```python
from build123d import *

# Parameters (mm, degrees)
BOSS_EXTRUDE1_DEPTH = 3.2
SKETCH2_R           = 6
CUT_EXTRUDE1_DEPTH  = 10


with BuildPart() as part:
    # Sketch1 → Boss-Extrude1 (new body)
    with BuildSketch(Plane.XY):
        with BuildLine():
            ThreePointArc((2.3749, 17.446481614), (2.211827147, 19.125468185), (1.72870442, 20.741692518))
            ThreePointArc((1.72870442, 20.741692518), (1.452377955, 21.089746522), (1.03228327, 21.234723622))
            ThreePointArc((1.03228327, 21.234723622), (0, 21.2598), (-1.03228327, 21.234723622))
            ThreePointArc((-1.03228327, 21.234723622), (-1.452377955, 21.089746522), (-1.72870442, 20.741692518))
            ThreePointArc((-1.72870442, 20.741692518), (-2.211827147, 19.125468185), (-2.3749, 17.446481614))
            ThreePointArc((-2.3749, 17.446481614), (-4.990435728, 13.711109477), (-9.395103266, 14.891336586))
            ThreePointArc((-9.395103266, 14.891336586), (-10.599256083, 16.07269371), (-12.00823854, 17.000248076))
            ThreePointArc((-12.00823854, 17.000248076), (-12.443641694, 17.089253684), (-12.858642377, 16.930280927))
            ThreePointArc((-12.858642377, 16.930280927), (-13.665536024, 16.285951652), (-14.440192102, 15.603203136))
            ThreePointArc((-14.440192102, 15.603203136), (-14.668813817, 15.222112575), (-14.656767369, 14.777868512))
            ThreePointArc((-14.656767369, 14.777868512), (-13.987971874, 13.22922354), (-13.033661162, 11.838223998))
            ThreePointArc((-13.033661162, 11.838223998), (-12.636226845, 7.295528971), (-16.769033299, 5.368369672))
            ThreePointArc((-16.769033299, 5.368369672), (-18.450829595, 5.49932722), (-20.12639323, 5.304198623))
            ThreePointArc((-20.12639323, 5.304198623), (-20.517143098, 5.092509122), (-20.732866347, 4.703971627))
            ThreePointArc((-20.732866347, 4.703971627), (-20.936815867, 3.691725528), (-21.091374564, 2.670770493))
            ThreePointArc((-21.091374564, 2.670770493), (-21.021548669, 2.23188298), (-20.726765974, 1.899315592))
            ThreePointArc((-20.726765974, 1.899315592), (-19.218989102, 1.142878174), (-17.593827413, 0.690729806))
            ThreePointArc((-17.593827413, 0.690729806), (-14.369386985, -2.533710622), (-16.296546284, -6.666517075))
            ThreePointArc((-16.296546284, -6.666517075), (-17.669054881, -7.647235594), (-18.827184848, -8.873744316))
            ThreePointArc((-18.827184848, -8.873744316), (-18.990445225, -9.287077056), (-18.905951734, -9.723378276))
            ThreePointArc((-18.905951734, -9.723378276), (-18.411526879, -10.6299), (-17.873668464, -11.511345346))
            ThreePointArc((-17.873668464, -11.511345346), (-17.538067269, -11.802669466), (-17.098480428, -11.867948202))
            ThreePointArc((-17.098480428, -11.867948202), (-15.457227734, -11.478232591), (-13.921646284, -10.779964538))
            ThreePointArc((-13.921646284, -10.779964538), (-9.378951257, -11.177398855), (-8.198724147, -15.582066393))
            ThreePointArc((-8.198724147, -15.582066393), (-8.619733019, -17.215571885), (-8.718527435, -18.899563668))
            ThreePointArc((-8.718527435, -18.899563668), (-8.577906975, -19.321136664), (-8.232732188, -19.60105142))
            ThreePointArc((-8.232732188, -19.60105142), (-7.271279843, -19.977677179), (-6.292674246, -20.307174764))
            ThreePointArc((-6.292674246, -20.307174764), (-5.848329281, -20.314621697), (-5.469625861, -20.082067135))
            ThreePointArc((-5.469625861, -20.082067135), (-4.462857721, -18.728550761), (-3.735372137, -17.206593669))
            ThreePointArc((-3.735372137, -17.206593669), (0, -14.591057941), (3.735372137, -17.206593669))
            ThreePointArc((3.735372137, -17.206593669), (4.462857721, -18.728550761), (5.469625861, -20.082067135))
            ThreePointArc((5.469625861, -20.082067135), (5.848329281, -20.314621697), (6.292674246, -20.307174764))
            ThreePointArc((6.292674246, -20.307174764), (7.271279843, -19.977677179), (8.232732188, -19.60105142))
            ThreePointArc((8.232732188, -19.60105142), (8.577906975, -19.321136664), (8.718527435, -18.899563668))
            ThreePointArc((8.718527435, -18.899563668), (8.619733019, -17.215571885), (8.198724147, -15.582066393))
            ThreePointArc((8.198724147, -15.582066393), (9.378951257, -11.177398855), (13.921646284, -10.779964538))
            ThreePointArc((13.921646284, -10.779964538), (15.457227734, -11.478232591), (17.098480428, -11.867948202))
            ThreePointArc((17.098480428, -11.867948202), (17.538067269, -11.802669466), (17.873668464, -11.511345346))
            ThreePointArc((17.873668464, -11.511345346), (18.411526879, -10.6299), (18.905951734, -9.723378276))
            ThreePointArc((18.905951734, -9.723378276), (18.990445225, -9.287077056), (18.827184848, -8.873744316))
            ThreePointArc((18.827184848, -8.873744316), (17.669054881, -7.647235594), (16.296546284, -6.666517075))
            ThreePointArc((16.296546284, -6.666517075), (14.369386985, -2.533710622), (17.593827413, 0.690729806))
            ThreePointArc((17.593827413, 0.690729806), (19.218989102, 1.142878174), (20.726765974, 1.899315592))
            ThreePointArc((20.726765974, 1.899315592), (21.021548669, 2.23188298), (21.091374564, 2.670770493))
            ThreePointArc((21.091374564, 2.670770493), (20.936815867, 3.691725528), (20.732866347, 4.703971627))
            ThreePointArc((20.732866347, 4.703971627), (20.517143098, 5.092509122), (20.12639323, 5.304198623))
            ThreePointArc((20.12639323, 5.304198623), (18.450829595, 5.49932722), (16.769033299, 5.368369672))
            ThreePointArc((16.769033299, 5.368369672), (12.636226845, 7.295528971), (13.033661162, 11.838223998))
            ThreePointArc((13.033661162, 11.838223998), (13.987971874, 13.22922354), (14.656767369, 14.777868512))
            ThreePointArc((14.656767369, 14.777868512), (14.668813817, 15.222112575), (14.440192102, 15.603203136))
            ThreePointArc((14.440192102, 15.603203136), (13.665536024, 16.285951652), (12.858642377, 16.930280927))
            ThreePointArc((12.858642377, 16.930280927), (12.443641694, 17.089253684), (12.00823854, 17.000248076))
            ThreePointArc((12.00823854, 17.000248076), (10.599256083, 16.07269371), (9.395103266, 14.891336586))
            ThreePointArc((9.395103266, 14.891336586), (4.990435728, 13.711109477), (2.3749, 17.446481614))
        make_face()
    extrude(amount=-BOSS_EXTRUDE1_DEPTH)

    # Sketch2 → Cut-Extrude1 (cut)
    with BuildSketch(Plane.XY):
        Circle(SKETCH2_R)
    extrude(amount=-CUT_EXTRUDE1_DEPTH, mode=Mode.SUBTRACT)


solid = part.part
```
For this review, take the finished solid that the model builds, in its own axes (mm). A direction names the side the tool comes from. Round coordinates to 2 decimals unless told otherwise and drop trailing zeros. Write each loop counter-clockwise with the first axis right and the second up, starting at its lowest first coordinate (ties: lowest second). Pieces come first, ordered by that corner, then holes. Notation, with made-up numbers: (59, 19) - (101, 19) arc R34 cw to (101, 51) - close; hole circle Ø3 at (71.25, -6.75). An arc over 180 degrees is marked (long way). Answer as a JSON object with one key per item and string values.
1. We need section A-A on x = 0. Give the boundary of the cut face in (y, z), then the cut area to 3 significant figures.
Response values:
{"outline": "(-14.59, -3.2) - (-6, -3.2) - (-6, 0) - (-14.59, 0) - close; (6, -3.2) - (21.26, -3.2) - (21.26, 0) - (6, 0) - close", "area": "76.3 mm2"}
2. For pin 1 Ø1.5 at (x, z) = (2, -1.5) entering from -Y, flat-tipped, find the tip position at first contact; note if it passes through.
Response values:
{"pin 1": "stops at y = -15.7"}
3. Tool access review of faces 1 (the face through (-17.65, -7.63, -1.58)), 2 (the face through (-9.431, -11.134, -1.578)), 3 (the face through (8.623, -17.239, -1.578)), 4 (the face through (10.62, 16.09, -1.58)), 5 (the face through (-2.207, 19.149, -1.578)): name each direction out of +Z, -Z, +X, -X, +Y, -Y from which nothing blocks a thin tool from reaching the whole face with its end or side.
Response values:
{"face 1": "+Z, -Z, -X", "face 2": "+Z, -Z", "face 3": "+Z, -Z, +X", "face 4": "+Z, -Z, +Y", "face 5": "+Z, -Z, -X, +Y"}
4. We need section B-B on y = -3.5. Give the boundary of the cut face in (x, z), then the cut area to 3 significant figures.
Response values:
{"outline": "(-14.32, -3.2) - (-4.87, -3.2) - (-4.87, 0) - (-14.32, 0) - close; (4.87, -3.2) - (14.32, -3.2) - (14.32, 0) - (4.87, 0) - close", "area": "60.4 mm2"}
5. We need section D-D on y = -13.5. Give the boundary of the cut face in (x, z).
Response values:
{"outline": "(-8.03, -3.2) - (8.03, -3.2) - (8.03, 0) - (-8.03, 0) - close"}
6. Draft analysis for pull direction X (two halves, no side actions). For faces 6 (the face through (20.94, 3.68, -1.58)), 7 (the face through (5.05, 13.69, -1.58)), 8 (the face through (-14.38, -2.47, -1.58)), 9 (the face through (-5, -4, 0)), state which applies: +X half, -X half, draft (parallel to the pull), parting line (faces both ways), or undercut.
Response values:
{"face 6": "+X half", "face 7": "undercut", "face 8": "-X half", "face 9": "draft"}
7. We need section C-C on y = 8. Give the boundary of the cut face in (x, z), then the cut area to 3 significant figures.
Response values:
{"outline": "(-12.32, -3.2) - (12.32, -3.2) - (12.32, 0) - (-12.32, 0) - close", "area": "78.8 mm2"}
8. To check wall thickness, follow line 1 along X through (y, z) = (15.5, -1.5); line 2 along Y through (x, z) = (-17, -2.35); line 3 along X through (y, z) = (9.5, -2.9). State the ranges of each line that lie inside material, in increasing order.
Response values:
{"line 1": "x = -14.53 to -9.96, -2.88 to 2.88, 9.96 to 14.53", "line 2": "y = -11.85 to -7.12, 0.54 to 5.41", "line 3": "x = -12.11 to 12.11"}
